Read the model definition and answer for the solid it produces. Units are mm, in the model's axes. A direction names the side the tool comes from. Coordinates: 2 decimals unless noted, no trailing zeros. Write each loop counter-clockwise with the first axis right and the second up, starting at its lowest first coordinate (ties: lowest second). Pieces come first, ordered by that corner, then holes. Notation, with made-up numbers: (11, -17.75) -> (51, -17.75) arc R34 cw to (51, 15.25) -> close; hole circle Ø3 at (-26.75, -10.5). An arc over 180 degrees is marked (long way). One line per item, written item: value. Start each with the question number.
1. Find section A-A, the plane x = -10.5. Write down the section's boundary in (y, z), and give its area (3 significant figures).
2. Find section D-D, the plane y = 1.75. Write down the section's boundary in (x, z).
3. Find section B-B, the plane z = 33. Write down the section's boundary in (x, y), and give its area (3 significant figures).
4. For faces 4 (the flat face through (4, 7, 25)), 5 (the flat face through (15, 3, 53.438)), determine the directions among +Z, -Z, +X, -X, +Y, -Y from which every point of the face is accessible in a straight line to the end or side of a thin tool.
5. Find section C-C, the plane x = -1. Write down the section's boundary in (y, z).
6. For a pull along X with two mould halves and no side action, classify faces 1 (the cylindrical face through (23.053, 3.451, 45.455)), 2 (the cylindrical face through (31.493, 3.549, -3.711)), 3 (the flat face through (4, 0, 25)) as pulls with the +X half, pulls with the -X half, needs draft (parallel to the pull), parting line crosses it, or undercut.
7. Consider line 1 along X through (y, z) = (5, 40); line 2 along X through (y, z) = (2.5, 42.5); line 3 along Z through (x, y) = (-8.5, 1). Determine where each line is inside the solid, lowest interval first.
```python
from build123d import *

# Parameters (mm, degrees)
SKETCH_1_W          = 60
SKETCH_1_H          = 60
EXTRUDE_1_DEPTH     = 7
SKETCH_2_R          = 4
SKETCH_2_R_2        = 11
CUT_EXTRUDE_1_DEPTH = 64.990752506
SKETCH_3_R          = 1.55
CUT_EXTRUDE_2_DEPTH = 64.990752506
FILLET_2_R          = 10
SKETCH_4_W          = 30.91835897
SKETCH_4_H          = 7
EXTRUDE_2_DEPTH     = 5
FILLET_3_R          = 10


with BuildPart() as part:
    # 草图1 → 凸台-拉伸1 (new body)
    with BuildSketch(Plane(origin=(0, 0, 0), x_dir=(1, 0, 0), z_dir=(0, 1, 0))):
        with Locations((4.5, -23.4375)):
            Rectangle(SKETCH_1_W, SKETCH_1_H)
    extrude(amount=EXTRUDE_1_DEPTH)

    # 草图2 → 切除-拉伸1 (cut, through all)
    with BuildSketch(Plane.XZ):
        with Locations(Location((19.679947821, 47.605596436, 0), (0, 0, 270))):
            Circle(SKETCH_2_R)
        with Locations(Location((-7.128568068, 39.524539832, 0), (0, 0, 270))):
            Circle(SKETCH_2_R_2)
    extrude(amount=-CUT_EXTRUDE_1_DEPTH, mode=Mode.SUBTRACT)

    # 草图3 → 切除-拉伸2 (cut, through all)
    with BuildSketch(Plane.XZ):
        with Locations(Location((-10.5, 2.024539832, 0), (0, 0, 270))):
            Circle(SKETCH_3_R)
        with Locations(Location((19.5, 2.024539832, 0), (0, 0, 270))):
            Circle(SKETCH_3_R)
    extrude(amount=-CUT_EXTRUDE_2_DEPTH, mode=Mode.SUBTRACT)

    # 圆角2
    fillet_2_edges = [part.edges().sort_by_distance(p)[0] for p in [
        (-25.5, 3.5, -6.5625),
        (34.5, 3.5, -6.5625),
        (34.5, 3.5, 53.4375),
    ]]
    fillet(fillet_2_edges, radius=FILLET_2_R)

    # 草图4 → 凸台-拉伸2 (add)
    with BuildSketch(Plane.XY.offset(53.4375)):
        with Locations((-10.040820515, 3.5)):
            Rectangle(SKETCH_4_W, SKETCH_4_H)
    extrude(amount=EXTRUDE_2_DEPTH)

    # 圆角3
    # the kernel refuses this fillet: 10 mm, written as the material it takes off along each edge
    with BuildSketch(Plane(origin=(5.41835897, -21.650635095, 58.4375), x_dir=(-1, 0, 0), z_dir=(0, 1, 0))) as fillet_3_piece_1:
        with BuildLine():
            CenterArc((8.660254038, -10), FILLET_3_R, 90, 60)
            Line((0, -5), (-0.173205081, -4.9))
            ThreePointArc((-0.173205081, -4.9), (-0.2, -2.5), (-0.2, 0))
            Line((-0.2, 0), (0, 0.2))
            Line((0, 0.2), (8.660254038, 0.2))
            Line((8.660254038, 0.2), (8.660254038, 0))
        make_face()
    extrude(amount=50.301270189, mode=Mode.SUBTRACT)
    with BuildSketch(Plane(origin=(-25.5, 32, 58.4375), x_dir=(0, 0, -1), z_dir=(0, -1, 0))) as fillet_3_piece_2:
        with BuildLine():
            CenterArc((FILLET_3_R, FILLET_3_R), FILLET_3_R, 180, 90)
            Line((0, FILLET_3_R), (-FILLET_3_R * 0.02, FILLET_3_R))
            Line((-FILLET_3_R * 0.02, FILLET_3_R), (-FILLET_3_R * 0.02, -FILLET_3_R * 0.02))
            Line((-FILLET_3_R * 0.02, -FILLET_3_R * 0.02), (FILLET_3_R, -FILLET_3_R * 0.02))
            Line((FILLET_3_R, -FILLET_3_R * 0.02), (FILLET_3_R, 0))
        make_face()
    extrude(amount=57, mode=Mode.SUBTRACT)


solid = part.part
```
Answer block:
1. outline: (0, -6.56) -> (7, -6.56) -> (7, 0.47) -> (0, 0.47) -> close; (0, 3.57) -> (7, 3.57) -> (7, 29.05) -> (0, 29.05) -> close; (0, 50) -> (7, 50) -> (7, 58.44) -> (0, 58.44) -> close
1. area: 287 mm2
2. outline: (-25.5, 3.44) arc R10 ccw to (-15.5, -6.56) -> (24.5, -6.56) arc R10 ccw to (34.5, 3.44) -> (34.5, 43.44) arc R10 ccw to (24.5, 53.44) -> (5.42, 53.44) arc R10 ccw to (-3.24, 58.44) -> (-15.5, 58.44) arc R10 ccw to (-25.5, 48.44) -> close; hole circle Ø22 at (-7.13, 39.52); hole circle Ø3.1 at (-10.5, 2.02); hole circle Ø8 at (19.68, 47.61); hole circle Ø3.1 at (19.5, 2.02)
3. outline: (-25.5, 0) -> (-15.98, 0) -> (-15.98, 7) -> (-25.5, 7) -> close; (1.73, 0) -> (34.5, 0) -> (34.5, 7) -> (1.73, 7) -> close
3. area: 296 mm2
4. face 4: +Z, -Z, +X, -X, +Y
4. face 5: +Z, +X, +Y, -Y
5. outline: (0, -6.56) -> (7, -6.56) -> (7, 30.39) -> (0, 30.39) -> close; (0, 48.66) -> (7, 48.66) -> (7, 58.18) -> (0, 58.18) -> close
6. face 1: undercut
6. face 2: pulls with the +X half
6. face 3: needs draft
7. line 1: x = -25.5 to -18.12, 3.86 to 34.5
7. line 2: x = -25.5 to -17.72, 3.46 to 34.5
7. line 3: z = -6.56 to 28.61, 50.44 to 58.44
